Answer from the drawing. Dimensions are ordinates in mm from the lowest x, y and z of the part. Coordinates: 2 decimals unless noted, no trailing zeros. Order: outer loops, then holes, each group sorted by start corner. A loop starts at its lowest first (then second) coordinate and runs counter-clockwise, first axis right, second up. Notation, with made-up numbers: (30, 45.25) -> (54, 45.25) arc R38 ccw to (54, 83.25) -> close; hole circle Ø5 at (20, 68). An arc over 180 degrees is marked (long way). Answer as a JSON object with one key per item and string values. Group by question number.
1) Section D-D on y = 0.25 is taken. Determine the outline of the cut face in (x, z).
2) Consider L1, parallel to Z at x = 7.75, y = 0.4; L2, parallel to X at y = 0.7, z = 37.5; L3, parallel to X at y = 1.1, z = 18.5. Determine where each line is inside the solid, lowest interval first.
3) Section C-C on z = 37.5 is taken. Determine the outline of the cut face in (x, y), and give its area (3 significant figures).
4) Section B-B on x = 40.5 is taken. Determine the outline of the cut face in (y, z).
5) Determine the mould class of the marked faces 1 and 2 for opening direction Y: released by +Y, released by -Y, zero draft, split by the parting line, or undercut.
6) Section A-A on z = 32 is taken. Determine the outline of the cut face in (x, y).
7) Given pin 1 (0.8 mm diameter, centred on y = 1, z = 19.5, fed in from -X); pin 2 (0.8 mm diameter, centred on x = 56.5, y = 0.5, fed in from +Z); pin 3 (2.5 mm diameter, centred on x = 7.75, z = 2.5, fed in from +Y), each flat-ended and moving along its own axis, determine where each tip first touches the part or whether it passes through.
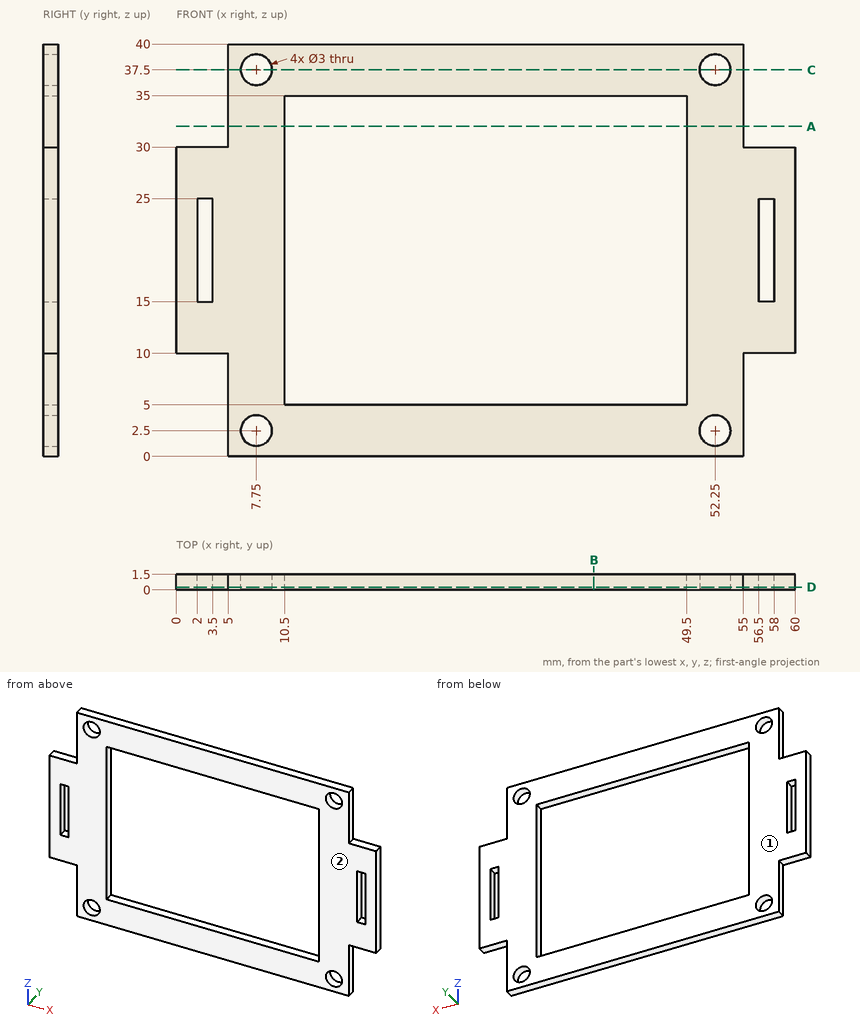
Worked answers:
{
 "1": {"outline": "(0, 10) -> (5, 10) -> (5, 0) -> (55, 0) -> (55, 10) -> (60, 10) -> (60, 30) -> (55, 30) -> (55, 40) -> (5, 40) -> (5, 30) -> (0, 30) -> close; hole (2, 15) -> (3.5, 15) -> (3.5, 25) -> (2, 25) -> close; hole circle Ø3 at (7.75, 2.5); hole circle Ø3 at (7.75, 37.5); hole (10.5, 5) -> (49.5, 5) -> (49.5, 35) -> (10.5, 35) -> close; hole circle Ø3 at (52.25, 2.5); hole circle Ø3 at (52.25, 37.5); hole (56.5, 15) -> (58, 15) -> (58, 25) -> (56.5, 25) -> close"},
 "2": {"L1": "z = 0 to 1, 4 to 36, 39 to 40", "L2": "x = 5 to 6.25, 9.25 to 50.75, 53.75 to 55", "L3": "x = 0 to 2, 3.5 to 10.5, 49.5 to 56.5, 58 to 60"},
 "3": {"outline": "(5, 0) -> (6.25, 0) -> (6.25, 1.5) -> (5, 1.5) -> close; (9.25, 0) -> (50.75, 0) -> (50.75, 1.5) -> (9.25, 1.5) -> close; (53.75, 0) -> (55, 0) -> (55, 1.5) -> (53.75, 1.5) -> close", "area": "66.0 mm²"},
 "4": {"outline": "(0, 0) -> (1.5, 0) -> (1.5, 5) -> (0, 5) -> close; (0, 35) -> (1.5, 35) -> (1.5, 40) -> (0, 40) -> close"},
 "5": {"face 1": "released by +Y", "face 2": "released by -Y"},
 "6": {"outline": "(5, 0) -> (10.5, 0) -> (10.5, 1.5) -> (5, 1.5) -> close; (49.5, 0) -> (55, 0) -> (55, 1.5) -> (49.5, 1.5) -> close"},
 "7": {"pin 1": "stops at x = 0", "pin 2": "stops at z = 30", "pin 3": "passes through"}
}
